```python
from build123d import *

# Parameters (mm, degrees)
CROQUIS1_W              = 7
CROQUIS1_H              = 7
SALIENTE_EXTRUIR1_DEPTH = 3
CROQUIS2_R              = 2.25
SALIENTE_EXTRUIR2_DEPTH = 2.5
CROQUIS3_W              = 7
CROQUIS3_H              = 9.5
SALIENTE_EXTRUIR3_DEPTH = 2
CROQUIS4_W              = 7
CROQUIS4_H              = 5
SALIENTE_EXTRUIR4_DEPTH = 20.02
CROQUIS5_W              = 29.52
CROQUIS5_H              = 5
SALIENTE_EXTRUIR5_DEPTH = 40.4
SALIENTE_EXTRUIR6_DEPTH = 7
CROQUIS7_R              = 2.25
CORTAR_EXTRUIR1_DEPTH   = 4.5
CROQUIS8_W              = 54.4
CROQUIS8_H              = 5
SALIENTE_EXTRUIR7_DEPTH = 0.48
CORTAR_EXTRUIR3_DEPTH   = 0.5
CROQUIS11_W             = 54.4
CROQUIS11_H             = 4.5
SALIENTE_EXTRUIR9_DEPTH = 10
CROQUIS12_R             = 1.5
CORTAR_EXTRUIR4_DEPTH   = 62.585797064
CHAFL_N1_SIZE           = 1
CROQUIS13_W             = 54.4
CROQUIS13_H             = 2.25
CORTAR_EXTRUIR5_DEPTH   = 69.707571635
REDONDEO1_R             = 10


with BuildPart() as part:
    # Croquis1 → Saliente-Extruir1 (new body)
    with BuildSketch(Plane(origin=(0, 0, 0), x_dir=(1, 0, 0), z_dir=(0, 1, 0))):
        Rectangle(CROQUIS1_W, CROQUIS1_H)
    extrude(amount=SALIENTE_EXTRUIR1_DEPTH)

    # Croquis2 → Saliente-Extruir2 (add)
    with BuildSketch(Plane.XY.offset(3.5)):
        Polygon((3.5, 3), (3.5, 23.02), (-3.5, 23.02), (-3.5, 3), (-3.5, 0), (3.5, 0), align=None)
        with Locations((0.5, 18.01)):
            Circle(CROQUIS2_R, mode=Mode.SUBTRACT)
    extrude(amount=SALIENTE_EXTRUIR2_DEPTH)

    # Croquis3 → Saliente-Extruir3 (add)
    with BuildSketch(Plane.XZ):
        with Locations((0, 1.25)):
            Rectangle(CROQUIS3_W, CROQUIS3_H)
    extrude(amount=SALIENTE_EXTRUIR3_DEPTH)

    # Croquis4 → Saliente-Extruir4 (add)
    with BuildSketch(Plane(origin=(0, 0, -3.5), x_dir=(-1, 0, 0), z_dir=(0, 0, -1))):
        with Locations((0, 0.5)):
            Rectangle(CROQUIS4_W, CROQUIS4_H)
    extrude(amount=SALIENTE_EXTRUIR4_DEPTH)

    # Croquis5 → Saliente-Extruir5 (add)
    with BuildSketch(Plane.ZY.offset(3.5)):
        with Locations((-8.76, 0.5)):
            Rectangle(CROQUIS5_W, CROQUIS5_H)
    extrude(amount=SALIENTE_EXTRUIR5_DEPTH)

    # Croquis6 → Saliente-Extruir6 (add)
    with BuildSketch(Plane.ZY.offset(43.9)):
        Polygon((6, 3), (6, 23.02), (3.5, 23.02), (3.5, 3), (-23.52, 3), (-23.52, -2), (6, -2), align=None)
    extrude(amount=SALIENTE_EXTRUIR6_DEPTH)

    # Croquis7 → Cortar-Extruir1 (cut)
    with BuildSketch(Plane.XY.offset(6)):
        with Locations((-47.9, 18.01)):
            Circle(CROQUIS7_R)
    extrude(amount=-CORTAR_EXTRUIR1_DEPTH, mode=Mode.SUBTRACT)

    # Croquis8 → Saliente-Extruir7 (add)
    with BuildSketch(Plane(origin=(0, 0, -23.52), x_dir=(-1, 0, 0), z_dir=(0, 0, -1))):
        with Locations((23.7, 0.5)):
            Rectangle(CROQUIS8_W, CROQUIS8_H)
    extrude(amount=SALIENTE_EXTRUIR7_DEPTH)

    # Croquis10 → Cortar-Extruir3 (cut)
    with BuildSketch(Plane(origin=(0, 3, 0), x_dir=(1, 0, 0), z_dir=(0, 1, 0))):
        Polygon((3.5, -3.5), (3.5, 24), (-50.9, 24), (-50.9, -3.5), (-43.9, -3.5), (-43.9, -6), (-3.5, -6), (-3.5, -3.5), align=None)
    extrude(amount=-CORTAR_EXTRUIR3_DEPTH, mode=Mode.SUBTRACT)

    # Croquis11 → Saliente-Extruir9 (add)
    with BuildSketch(Plane.XY.offset(6)):
        with Locations((-23.7, 0.25)):
            Rectangle(CROQUIS11_W, CROQUIS11_H)
    extrude(amount=SALIENTE_EXTRUIR9_DEPTH)

    # Croquis12 → Cortar-Extruir4 (cut, through all)
    with BuildSketch(Plane.XZ.offset(2)):
        with Locations(Location((-0.5, 12, 0), (0, 0, 270))):
            Circle(CROQUIS12_R)
        with Locations(Location((-0.5, -20, 0), (0, 0, 270))):
            Circle(CROQUIS12_R)
    extrude(amount=-CORTAR_EXTRUIR4_DEPTH, mode=Mode.SUBTRACT)

    # Chaflán1
    chafl_n1_edges = [part.edges().sort_by_distance(p)[0] for p in [
        (-0.5, 2.5, 13.5),
        (-0.5, 2.5, -18.5),
    ]]
    chamfer(chafl_n1_edges, length=CHAFL_N1_SIZE)

    # Croquis13 → Cortar-Extruir5 (cut, through all)
    with BuildSketch(Plane.XY.offset(16)):
        with Locations((-23.7, -0.875)):
            Rectangle(CROQUIS13_W, CROQUIS13_H)
    extrude(amount=-CORTAR_EXTRUIR5_DEPTH, mode=Mode.SUBTRACT)

    # Redondeo1
    redondeo1_edges = [part.edges().sort_by_distance(p)[0] for p in [
        (0, 2.5, 3.5),
        (-47.4, 2.5, 3.5),
    ]]
    fillet(redondeo1_edges, radius=REDONDEO1_R)


solid = part.part
```
Part model, mm, in its own coordinate system. A direction names the side the tool comes from. Round coordinates to 2 decimals unless told otherwise and drop trailing zeros. Loops run counter-clockwise (first coordinate to the right, second up) from the corner with the lowest first, then second, coordinate; pieces in that order, holes last. Notation, with made-up numbers: (46.5, 9.25) -> (83.5, 9.25) arc R26 cw to (83.5, 35.25) -> close; hole circle Ø11 at (65.5, -10.5). An arc over 180 degrees is marked (long way). Use a Markdown table: item, result.
1) Pull direction X, two halves, no side cores. Call faces 4 (the flat face through (-24, 1, 16)), 5 (the flat face through (3.5, 3.1, -2.6)), 6 (the flat face through (-43.9, 11, 4)): pulls with the +X half, pulls with the -X half, needs draft (parallel to the pull), parting line crosses it, or undercut.
The answers:
| item | result |
|---|---|
| face 4 | needs draft |
| face 5 | pulls with the +X half |
| face 6 | undercut |
2) Cut at D-D, the plane x = -0.5. List the corners of the cut face in (y, z).
The answers:
| item | result |
|---|---|
| outline | (0.25, -24) -> (2.5, -24) -> (2.5, -22.5) -> (1.5, -21.5) -> (0.25, -21.5) -> close; (0.25, -18.5) -> (1.5, -18.5) -> (2.5, -17.5) -> (2.5, -6.5) arc R10 cw to (12.5, 3.5) -> (15.99, 3.5) -> (15.99, 6) -> (2.5, 6) -> (2.5, 9.5) -> (1.5, 10.5) -> (0.25, 10.5) -> close; (0.25, 13.5) -> (1.5, 13.5) -> (2.5, 14.5) -> (2.5, 16) -> (0.25, 16) -> close; (20.03, 3.5) -> (23.02, 3.5) -> (23.02, 6) -> (20.03, 6) -> close |
3) Probe line 1 (X direction, y = 7.5, z = 5); line 2 (Y direction, x = 0.5, z = 4.25); line 3 (Y direction, x = -27.5, z = -21). List the from-to ranges inside material, lowest first. Write a range as [from, to].
The answers:
| item | result |
|---|---|
| line 1 | x = [-50.9, -43.9], [-3.5, 3.5] |
| line 2 | y = [0.25, 15.76], [20.26, 23.02] |
| line 3 | y = [0.25, 2.5] |
4) Cut at A-A, the plane x = -47.9. List the corners of the cut face in (y, z), and give its area (3 significant figures).
The answers:
| item | result |
|---|---|
| outline | (0.25, -24) -> (2.5, -24) -> (2.5, -6.5) arc R10 cw to (12.5, 3.5) -> (15.76, 3.5) -> (15.76, 6) -> (2.5, 6) -> (2.5, 16) -> (0.25, 16) -> close; (20.26, 3.5) -> (23.02, 3.5) -> (23.02, 6) -> (20.26, 6) -> close |
| area | 152 mm2 |
5) Tool access for faces 1 (the cylindrical face through (0.012, 15.814, 4.732)), 2 (the flat face through (-3.5, 9.7, 3.5)), 3 (the flat face through (-45.89, 16.66, 3.5)): list every direction of +Z, -Z, +X, -X, +Y, -Y with a clear straight run to the whole face (end or side of a thin tool).
The answers:
| item | result |
|---|---|
| face 1 | +Z, -Z |
| face 2 | +Z, -Z, +Y |
| face 3 | -Z, +X, -X, +Y |
6) Cut at C-C, the plane z = -20. List the corners of the cut face in (x, y).
The answers:
| item | result |
|---|---|
| outline | (-50.9, 0.25) -> (-2, 0.25) -> (-2, 1.5) -> (-3, 2.5) -> (-50.9, 2.5) -> close; (1, 0.25) -> (3.5, 0.25) -> (3.5, 2.5) -> (2, 2.5) -> (1, 1.5) -> close |
7) Cut at B-B, the plane y = 18.01. List the corners of the cut face in (x, z), and give its area (3 significant figures).
The answers:
| item | result |
|---|---|
| outline | (-50.9, 3.5) -> (-50.15, 3.5) -> (-50.15, 6) -> (-50.9, 6) -> close; (-45.65, 3.5) -> (-43.9, 3.5) -> (-43.9, 6) -> (-45.65, 6) -> close; (-3.5, 3.5) -> (-1.75, 3.5) -> (-1.75, 6) -> (-3.5, 6) -> close; (2.75, 3.5) -> (3.5, 3.5) -> (3.5, 6) -> (2.75, 6) -> close |
| area | 12.5 mm2 |
8) Drop flat-ended pins along their axis: pin 1 Ø7 at (x, y) = (-47.9, 18.01) entering from -Z; pin 2 Ø1.8 at (x, z) = (-0.5, -20) entering from -Y; pin 3 Ø7.5 at (x, y) = (0, 18) entering from +Z; pin 4 Ø20 at (x, z) = (-28, -13) entering from +Y. Give the stop position or say it passes through.
The answers:
| item | result |
|---|---|
| pin 1 | stops at z = 3.5 |
| pin 2 | passes through |
| pin 3 | stops at z = 6 |
| pin 4 | stops at y = 2.5 |
